Design review of the part built by this model. Coordinates are the model's own, in mm. A direction names the side the tool comes from. Coordinates: 2 decimals unless noted, no trailing zeros. Write each loop counter-clockwise with the first axis right and the second up, starting at its lowest first coordinate (ties: lowest second). Pieces come first, ordered by that corner, then holes. Notation, with made-up numbers: M -6.75,81.5 L 10.25,81.5 A25 ccw 10.25,97.5 Z; hole C 57.25,14 d3. An arc over 180 degrees is marked long. One line per question, with ' | ' between items.
Autodesk Inventor part; units mm, degrees
ref_plane "YZ Plane" through (0, 0, 0) normal (1, 0, 0) x (0, 1, 0)
ref_plane "XZ Plane" through (0, 0, 0) normal (0, 1, 0) x (-1, 0, 0)
ref_plane "XY Plane" through (0, 0, 0) normal (0, 0, 1) x (1, 0, 0)
sketch "Sketch1" plane through (0, 0, 0) normal (0, 1, 0) x (-1, 0, 0)
  line L0 (0, 0) -> (21.25, 0)
  line L1 (21.25, 0) -> (21.25, -6.5)
  line L2 (21.25, -6.5) -> (0, -6.5) construction
  line L3 (0, -6.5) -> (0, 0)
  line L4 (0, -6.5) -> (20, -6.5) construction
  line L5 (20, -6.5) -> (20, -8.5) construction
  line L6 (20, -8.5) -> (0, -8.5)
  line L7 (0, -8.5) -> (0, -6.5)
  line L8 (21.25, -6.5) -> (20, -8.5)
  line L9 (21.25, -1.6) -> (20.75, -1.6)
  line L10 (20.75, -1.6) -> (20.75, -2.6)
  line L11 (20.75, -2.6) -> (21.25, -2.6) construction
  line L12 (21.25, -2.6) -> (21.25, -1.6)
  line L13 (21.25, -3.4) -> (20.75, -3.4)
  line L14 (20.75, -3.4) -> (20.75, -4.4)
  line L15 (20.75, -4.4) -> (21.25, -4.4)
  line L16 (21.25, -4.4) -> (21.25, -3.4)
  line L17 (0, 0) -> (20, 0) construction
  line L18 (20, 0) -> (20, -4.75)
  line L19 (20, -4.75) -> (5, -4.75)
  line L20 (0, -4.75) -> (0, 0)
  line L21 (5, -4.75) -> (8, -4.75)
  line L22 (8, -4.75) -> (8, 0) construction
  line L23 (8, 0) -> (0, 0)
  line L24 (0, 0) -> (0, -4.75)
  line L25 (8, -4.75) -> (7, 0)
  line L26 (0, -8.5) -> (5, -8.5)
  line L27 (5, -8.5) -> (5, -4.5)
  line L28 (5, -4.5) -> (0, -4.5)
  line L29 (0, -4.5) -> (0, -8.5)
  line L30 (0, -4.5) -> (4, -4.5)
  line L31 (4, -4.5) -> (4, 13.5)
  line L32 (4, 13.5) -> (0, 13.5)
  line L33 (0, 13.5) -> (0, -4.5)
  line L34 (0, 13.5) -> (5, 13.5)
  line L35 (5, 13.5) -> (5, 17.5)
  line L36 (5, 17.5) -> (0, 17.5)
  line L37 (0, 17.5) -> (0, 13.5)
  line L38 (0, 17.5) -> (6.75, 17.5)
  line L39 (6.75, 17.5) -> (6.75, 0)
  line L40 (6.75, 0) -> (0, 0)
  line L41 (0, 0) -> (0, 17.5)
  point P0 (6.75, 0)
  dimension "d0" = 21.25
  dimension "d1" = 6.5
  dimension "d2" = 20
  dimension "d3" = 2
  dimension "d4" = 1.6
  dimension "d5" = 1
  dimension "d6" = 1
  dimension "d7" = 0.8
  dimension "d8" = 0.5
  dimension "d9" = 1.25
  dimension "d10" = 3.75
  dimension "d11" = 8
  dimension "d12" = 7
  dimension "d13" = 5
  dimension "d14" = 4
  dimension "d15" = 4
  dimension "d16" = 18
  dimension "d17" = 5
  dimension "d18" = 4
  dimension "d19" = 6.75
revolve "Revolution1" add sketch "Sketch1" angle 360 about axis through (0, 0, 13.5) along (0, 0, -1) contours L0 L25 L19 L27 L28 L31 | L0 L31 L34 L35 L38 L39 | L19 L18 L0 L1 L13 L14 L15 L8 L6 L27
sketch "Sketch2" plane through (0, 0, -8.5) normal (0, 0, -1) x (-1, 0, 0)
  circle A0 centre (0, 0) radius 12.5 construction
  circle A1 centre (0, 12.5) radius 1.5
  line L0 (0, 17.5) -> (0, 0) construction
  arc A2 (11.782, 5.494) -> (5.494, 11.782) centre (0, 0) ccw construction
  arc A3 (14.9541, 6.9732) -> (6.9732, 14.9541) centre (0, 0) ccw
  arc A4 (8.6099, 4.0149) -> (4.0149, 8.6099) centre (0, 0) ccw
  arc A5 (8.6099, 4.0149) -> (14.9541, 6.9732) centre (11.782, 5.494) ccw
  arc A6 (6.9732, 14.9541) -> (4.0149, 8.6099) centre (5.494, 11.782) ccw
  line L1 (5.494, 11.782) -> (0, 0) construction
  line L2 (0, 0) -> (11.782, 5.494) construction
  circle A7 centre (0, 0) radius 17.5 construction
  circle A8 centre (0, 27.5) radius 10
  circle A9 centre (-12.5, 0) radius 1.5
  arc A10 (-14.9541, 6.9732) -> (-8.6099, 4.0149) centre (-11.782, 5.494) ccw
  arc A11 (-4.0149, 8.6099) -> (-8.6099, 4.0149) centre (0, 0) ccw
  arc A12 (-6.9732, 14.9541) -> (-14.9541, 6.9732) centre (0, 0) ccw
  arc A13 (-4.0149, 8.6099) -> (-6.9732, 14.9541) centre (-5.494, 11.782) ccw
  circle A14 centre (0, -12.5) radius 1.5
  arc A15 (-6.9732, -14.9541) -> (-4.0149, -8.6099) centre (-5.494, -11.782) ccw
  arc A16 (-8.6099, -4.0149) -> (-4.0149, -8.6099) centre (0, 0) ccw
  arc A17 (-14.9541, -6.9732) -> (-6.9732, -14.9541) centre (0, 0) ccw
  arc A18 (-8.6099, -4.0149) -> (-14.9541, -6.9732) centre (-11.782, -5.494) ccw
  circle A19 centre (12.5, 0) radius 1.5
  arc A20 (14.9541, -6.9732) -> (8.6099, -4.0149) centre (11.782, -5.494) ccw
  arc A21 (4.0149, -8.6099) -> (8.6099, -4.0149) centre (0, 0) ccw
  arc A22 (6.9732, -14.9541) -> (14.9541, -6.9732) centre (0, 0) ccw
  arc A23 (4.0149, -8.6099) -> (6.9732, -14.9541) centre (5.494, -11.782) ccw
  circle A24 centre (-19.4454, 19.4454) radius 10
  circle A25 centre (-27.5, 0) radius 10
  circle A26 centre (-19.4454, -19.4454) radius 10
  circle A27 centre (0, -27.5) radius 10
  circle A28 centre (19.4454, -19.4454) radius 10
  circle A29 centre (27.5, 0) radius 10
  circle A30 centre (19.4454, 19.4454) radius 10
  point P0 (-12.3744, 12.3744)
  point P1 (-17.5, 0)
  point P2 (-12.3744, -12.3744)
  point P3 (0, -17.5)
  point P4 (12.3744, -12.3744)
  point P5 (17.5, 0)
  point P6 (12.3744, 12.3744)
  dimension "d21" = 25
  dimension "d27" = 20
  dimension "d22" = 3
  dimension "d23" = 7
  dimension "d24" = 25
  dimension "d25" = 0.5
  dimension "d26" = 40
  dimension "d28" = 35
  dimension "d31" = 360
  dimension "d35" = 360
extrude "Extrusion1" cut sketch "Sketch2" against normal blind 6
properties part number "BASE" material "Stainless Steel"
1. To check wall thickness, follow line 1 along Y through (x, z) = (0, 9.25); line 2 along Y through (x, z) = (12.5, -6); line 3 along Y through (x, z) = (0, 14.55). State the ranges of each line that lie inside material, in increasing order. Write a range as [from, to].
Answer sheet:
line 1: [-6.75, -4], [4, 6.75] | line 2: [-12.25, -10.77], [-2.07, -1.5], [1.5, 2.07], [10.77, 12.25] | line 3: [-6.75, -5], [5, 6.75]
2. Tool access review of faces 5 (the face through (-19.4, 8, -3.4)), 6 (the face through (-18.475, -7.66, -1.88)), 7 (the face through (19.4, 8, -3.4)), 8 (the face through (-0.1, -17.5, -6.2)): name each direction out of +Z, -Z, +X, -X, +Y, -Y from which nothing blocks a thin tool from reaching the whole face with its end or side.
Answer sheet:
face 5: -X, +Y | face 6: +Z | face 7: +X, +Y | face 8: -Z, -Y
3. Take a section at D-D (z = 9.5). Write out the cut boundary in (x, y).
Answer sheet:
outline: C 0,0 d13.5; hole C 0,0 d8
4. Insertion check: pin 1 Ø1.4 at (x, y) = (8, -19.5) entering from +Z; pin 2 Ø0.6 at (x, y) = (20, -3) entering from -Z; pin 3 Ø2 at (y, z) = (-2.5, 8.5) entering from +X. Each pin has a flat end and moves straight along its axis. Give the tip position at first contact, or say it passes through.
Answer sheet:
pin 1: z = 0 | pin 2: z = -2.5 | pin 3: x = 6.58
5. Take a section at B-B (x = 12.5). Write out the cut boundary in (y, z).
Answer sheet:
outline: M -17.18,-2.5 L -15.61,-2.5 L -15.61,0 L -17.18,0 Z; M -12.25,-8.5 L -10.77,-8.5 L -10.77,-4.75 L -12.25,-4.75 Z; M -2.07,-8.5 L -1.5,-8.5 L -1.5,-4.75 L -2.07,-4.75 Z; M 1.5,-8.5 L 2.07,-8.5 L 2.07,-4.75 L 1.5,-4.75 Z; M 10.77,-8.5 L 12.25,-8.5 L 12.25,-4.75 L 10.77,-4.75 Z; M 15.61,-2.5 L 17.18,-2.5 L 17.18,0 L 15.61,0 Z
6. Draft analysis for pull direction X (two halves, no side actions). For faces 1 (the face through (12.45, 12.3, -6.21)), 2 (the face through (0.867, 3.905, 4.626)), 3 (the face through (-8.151, 19.625, -5.465)), 4 (the face through (14, -15, -2.5)), state which applies: pulls with the +X half, pulls with the -X half, needs draft (parallel to the pull), parting line crosses it, or undercut.
Answer sheet:
face 1: pulls with the +X half | face 2: undercut | face 3: pulls with the -X half | face 4: needs draft
7. Take a section at A-A (z = -0.75). Write out the cut boundary in (x, y).
Answer sheet:
outline: C 0,0 d42.5; C 0,0 d14.32; hole C 0,0 d40; hole C 0,0 d8
